The listing builds one solid part. Answer for the finished solid, in the listing's coordinates (mm). Face numbers are marked on the shaded views. Give positions to 0.01 mm unless a question says otherwise; leave off trailing zeros. Order: outer loops, then holes, each group sorted by start corner. A loop starts at its lowest first (then second) coordinate and runs counter-clockwise, first axis right, second up. Notation, with made-up numbers: (-12.5, 17) - (2.5, 17) arc R18 cw to (2.5, 42) - close; hole circle Ø10 at (89, -15). An arc over 180 degrees is marked (long way). Answer as a JSON object with one key per item and string values. Group by question number.
Q1. The mould has two halves that part along Y. Classify the marked faces 1, 2 and 3: released by +Y, released by -Y, zero draft, split by the parting line, or undercut.
Q2. Consider line 1 (Y direction, x = 0, z = 2.3); line 2 (X direction, y = 0.5, z = 3); line 3 (Y direction, x = 1.25, z = 0.8). Determine where each line is inside the solid, lowest interval first.
Q3. Given pin 1 (3.5 mm diameter, centred on x = 0, y = 0, fed in from +Z); pin 2 (1.4 mm diameter, centred on x = 0.5, y = 0.5, fed in from -Z); pin 3 (1.5 mm diameter, centred on x = -0.5, z = 0.5, fed in from -Y); pin 4 (2 mm diameter, centred on y = -2.5, z = 0.5, fed in from +X), each flat-ended and moving along its own axis, determine where each tip first touches the part or whether it passes through.
Q4. A cutting plane is placed at A-A, the plane z = 2.5. Give the vertices of the cut face in (x, y), and give its area (3 significant figures).
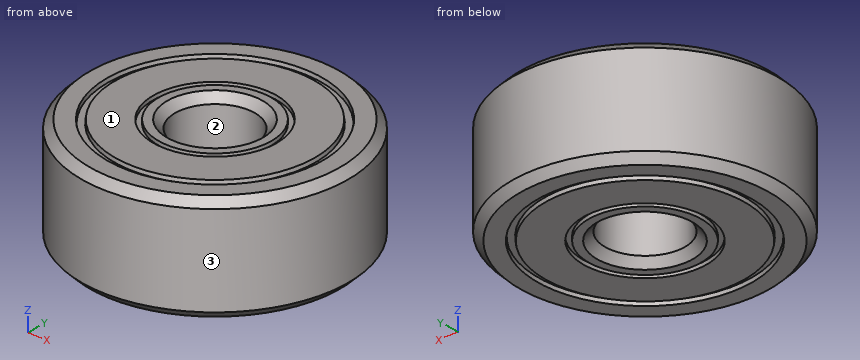
from build123d import *

# Parameters (mm, degrees)
CROQUIS1_R              = 5
CROQUIS1_R_2            = 1.5
SALIENTE_EXTRUIR1_DEPTH = 4
CHAFL_N1_SIZE           = 0.3
CROQUIS2_W              = 1
CROQUIS2_H              = 0.2


with BuildPart() as part:
    # Croquis1 → Saliente-Extruir1 (new body)
    with BuildSketch(Plane.XY):
        Circle(CROQUIS1_R)
        Circle(CROQUIS1_R_2, mode=Mode.SUBTRACT)
    extrude(amount=SALIENTE_EXTRUIR1_DEPTH)

    # Chaflán1
    chafl_n1_edges = [part.edges().sort_by_distance(p)[0] for p in [
        (-5, 0, 0),
        (-5, 0, 4),
        (-1.5, 0, 0),
        (-1.5, 0, 4),
    ]]
    chamfer(chafl_n1_edges, length=CHAFL_N1_SIZE)

    # Croquis2 → Cortar-Revolución1 (revolve, cut)
    with BuildSketch(Plane(origin=(0, 0, 0), x_dir=(0, 0, -1), z_dir=(1, 0, 0))):
        Polygon((-4.85, 4.150466692), (-3.85, 4.025466692), (-3.85, 3.775466692), (-4.85, 3.650466692), align=None)
        Polygon((0.85, 3.650466692), (0.85, 4.150466692), (-0.15, 4.025466692), (-0.15, 3.775466692), align=None)
        with Locations((-4.35, 2.220733596)):
            Rectangle(CROQUIS2_W, CROQUIS2_H)
        with Locations((0.35, 2.220733596)):
            Rectangle(CROQUIS2_W, CROQUIS2_H)
    revolve(axis=Axis((0, 0, 12.411349243), (0, 0, -1)), mode=Mode.SUBTRACT)


solid = part.part
Reply:
{
 "1": {"face 1": "zero draft", "face 2": "undercut", "face 3": "split by the parting line"},
 "2": {"line 1": "y = -5 to -1.5, 1.5 to 5", "line 2": "x = -4.97 to -1.41, 1.41 to 4.97", "line 3": "y = -4.84 to -0.83, 0.83 to 4.84"},
 "3": {"pin 1": "stops at z = 3.95", "pin 2": "passes through", "pin 3": "stops at y = -5", "pin 4": "stops at x = 4.77"},
 "4": {"outline": "circle Ø10 at (0, 0); hole circle Ø3 at (0, 0)", "area": "71.5 mm^2"}
}
